CAD build for the part. Positions are in the model's coordinates, mm. A direction names the side the tool comes from. Give positions to 0.01 mm unless a question says otherwise; leave off trailing zeros. Loops run counter-clockwise (first coordinate to the right, second up) from the corner with the lowest first, then second, coordinate; pieces in that order, holes last.
```python
from build123d import *

# Parameters (mm, degrees)
SKETCH1_R                = 72.63
BOSS_EXTRUDE1_DEPTH      = 13
BOSS_EXTRUDE2_DEPTH      = 5
SKETCH4_R                = 85.63
BOSS_EXTRUDE3_DEPTH      = 3.5
BOSS_EXTRUDE3_DEPTH_BACK = 5
CUT_EXTRUDE1_DEPTH       = 6
FILLET1_R                = 50
FILLET2_R                = 5
SKETCH8_R                = 2.4
CUT_EXTRUDE2_DEPTH       = 9.5
SKETCH10_OUTSIDE_W       = 230.742
SKETCH10_OUTSIDE_H       = 289.594
SKETCH10_OUTSIDE_R       = 60
CUT_EXTRUDE3_DEPTH       = 19
SKETCH11_R               = 2.4
CUT_EXTRUDE4_DEPTH       = 19


with BuildPart() as part:
    # Sketch1 → Boss-Extrude1 (new body)
    with BuildSketch(Plane(origin=(0, 0, 0), x_dir=(1, 0, 0), z_dir=(0, 1, 0))):
        Circle(SKETCH1_R)
    extrude(amount=BOSS_EXTRUDE1_DEPTH)

    # Sketch2 → Boss-Extrude2 (add)
    with BuildSketch(Plane(origin=(0, 13, 0), x_dir=(1, 0, 0), z_dir=(0, 1, 0))):
        with BuildLine():
            Line((-21.15, -69.482331567), (-21.15, -144.482331567))
            Line((-21.15, -144.482331567), (21.15, -144.482331567))
            Line((21.15, -144.482331567), (21.15, -69.482331567))
            ThreePointArc((21.15, -69.482331567), (0, 72.63), (-21.15, -69.482331567))
        make_face()
    extrude(amount=BOSS_EXTRUDE2_DEPTH)

    # Sketch4 → Boss-Extrude3 (add, two sides)
    with BuildSketch(Plane.XZ.offset(-13)) as boss_extrude3_sk:
        Circle(SKETCH4_R)
    extrude(amount=BOSS_EXTRUDE3_DEPTH)
    extrude(boss_extrude3_sk.sketch, amount=-BOSS_EXTRUDE3_DEPTH_BACK)

    # Sketch5 → Cut-Extrude1 (cut, through all)
    with BuildSketch(Plane.XZ.offset(-13)):
        with BuildLine():
            Line((11.25, 123.332331567), (11.25, 119.332331567))
            ThreePointArc((11.25, 119.332331567), (0, 108.082331567), (-11.25, 119.332331567))
            Line((-11.25, 119.332331567), (-11.25, 123.332331567))
            ThreePointArc((-11.25, 123.332331567), (0, 134.582331567), (11.25, 123.332331567))
        make_face()
        with BuildLine():
            Line((17.05, 107.832331567), (17.05, 103.832331567))
            ThreePointArc((17.05, 103.832331567), (15.5, 102.282331567), (13.95, 103.832331567))
            Line((13.95, 103.832331567), (13.95, 107.832331567))
            ThreePointArc((13.95, 107.832331567), (15.5, 109.382331567), (17.05, 107.832331567))
        make_face()
        with BuildLine():
            Line((17.05, 138.832331567), (17.05, 134.832331567))
            ThreePointArc((17.05, 134.832331567), (15.5, 133.282331567), (13.95, 134.832331567))
            Line((13.95, 134.832331567), (13.95, 138.832331567))
            ThreePointArc((13.95, 138.832331567), (15.5, 140.382331567), (17.05, 138.832331567))
        make_face()
        with BuildLine():
            Line((-13.95, 138.832331567), (-13.95, 134.832331567))
            ThreePointArc((-13.95, 134.832331567), (-15.5, 133.282331567), (-17.05, 134.832331567))
            Line((-17.05, 134.832331567), (-17.05, 138.832331567))
            ThreePointArc((-17.05, 138.832331567), (-15.5, 140.382331567), (-13.95, 138.832331567))
        make_face()
        with BuildLine():
            Line((-13.95, 107.832331567), (-13.95, 103.832331567))
            ThreePointArc((-13.95, 103.832331567), (-15.5, 102.282331567), (-17.05, 103.832331567))
            Line((-17.05, 103.832331567), (-17.05, 107.832331567))
            ThreePointArc((-17.05, 107.832331567), (-15.5, 109.382331567), (-13.95, 107.832331567))
        make_face()
    extrude(amount=-CUT_EXTRUDE1_DEPTH, mode=Mode.SUBTRACT)

    # Fillet1
    fillet1_edges = [part.edges().sort_by_distance(p)[0] for p in [
        (-21.15, 15.5, 82.976951017),
        (21.15, 15.5, 82.976951017),
    ]]
    fillet(fillet1_edges, radius=FILLET1_R)

    # Fillet2
    fillet2_edges = [part.edges().sort_by_distance(p)[0] for p in [
        (-21.15, 15.5, 144.482331567),
        (21.15, 15.5, 144.482331567),
    ]]
    fillet(fillet2_edges, radius=FILLET2_R)

    # Sketch8 → Cut-Extrude2 (cut, through all)
    with BuildSketch(Plane.XZ.offset(-9.5)):
        with Locations((0, 78.7622)):
            Circle(SKETCH8_R)
    extrude(amount=-CUT_EXTRUDE2_DEPTH, mode=Mode.SUBTRACT)

    # Sketch10 outside → Cut-Extrude3 (cut, through all)
    with BuildSketch(Plane.XZ):
        with Locations((0, 29.426)):
            Rectangle(SKETCH10_OUTSIDE_W, SKETCH10_OUTSIDE_H)
        with Locations((0, 121.332331567)):
            Circle(SKETCH10_OUTSIDE_R, mode=Mode.SUBTRACT)
    extrude(amount=-CUT_EXTRUDE3_DEPTH, mode=Mode.SUBTRACT)

    # Sketch11 → Cut-Extrude4 (cut, through all)
    with BuildSketch(Plane.XZ):
        with Locations((-12.636876971, 67.569177035)):
            Circle(SKETCH11_R)
        with Locations((12.636876971, 67.569177035)):
            Circle(SKETCH11_R)
    extrude(amount=-CUT_EXTRUDE4_DEPTH, mode=Mode.SUBTRACT)


solid = part.part
```
1. Saw through at C-C, the plane x = -25. List the corners of the cut face in (y, z), and give its area (3 significant figures).
Responses:
outline: (0, 66.79) - (18, 66.79) - (18, 96.23) - (13, 96.23) - (13, 81.9) - (9.5, 81.9) - (9.5, 68.19) - (0, 68.19) - close
area: 213 mm2
2. Pull direction Z, two halves, no side cores. Call faces 1 (the face through (19.6, 15.5, 143.1)), 2 (the face through (-1, 9.5, 75)), 3 (the face through (-15.534, 15.465, 109.382)): released by +Z, released by -Z, zero draft, split by the parting line, or undercut.
Responses:
face 1: released by +Z
face 2: zero draft
face 3: undercut
3. Saw through at B-B, the plane z = 125. List the corners of the cut face in (x, y), and give its area (3 significant figures).
Responses:
outline: (-21.15, 13) - (-11.13, 13) - (-11.13, 18) - (-21.15, 18) - close; (11.13, 13) - (21.15, 13) - (21.15, 18) - (11.13, 18) - close
area: 100 mm2
4. Saw through at A-A, the plane x = 0. List the corners of the cut face in (y, z).
Responses:
outline: (0, 61.33) - (18, 61.33) - (18, 76.36) - (9.5, 76.36) - (9.5, 72.63) - (0, 72.63) - close; (9.5, 81.16) - (18, 81.16) - (18, 108.08) - (13, 108.08) - (13, 85.63) - (9.5, 85.63) - close; (13, 134.58) - (18, 134.58) - (18, 144.48) - (13, 144.48) - close
5. Saw through at D-D, the plane y = 11.5. List the corners of the cut face in (x, z).
Responses:
outline: (-39.36, 76.05) arc R60 ccw to (39.36, 76.05) arc R85.63 ccw to start; hole circle Ø4.8 at (-12.64, 67.57); hole circle Ø4.8 at (0, 78.76); hole circle Ø4.8 at (12.64, 67.57)
6. Drop flat-ended pins along their axis: pin 1 (14.5 mm diameter, centred on x = 5, z = 78.5, fed in from -Y); pin 2 (4.5 mm diameter, centred on y = 15.5, z = 137.5, fed in from -X); pin 3 (1.2 mm diameter, centred on y = 15.5, z = 105.5, fed in from -X); pin 4 (1.5 mm diameter, centred on x = -23.5, z = 135, fed in from +Y). Give the stop position or say it passes through.
Responses:
pin 1: stops at y = 0
pin 2: stops at x = -21.15
pin 3: stops at x = -22.28
pin 4: passes through
7. Probe line 1 along Z through (x, y) = (0, 12.5); line 2 along X through (y, z) = (16.25, 128); line 3 along Y through (x, z) = (35.5, 73). List the from-to ranges inside material, lowest first.
Responses:
line 1: z = 61.33 to 76.36, 81.16 to 85.63
line 2: x = -21.15 to -10.24, 10.24 to 21.15
line 3: y = 9.5 to 18
8. Tool access for faces 4 (the face through (0, 15, 144.482)), 5 (the face through (-21.15, 15, 127)), 6 (the face through (13.95, 15, 106)), 7 (the face through (21.15, 15, 128)): list every direction of +Z, -Z, +X, -X, +Y, -Y with a clear straight run to the whole face (end or side of a thin tool).
Responses:
face 4: +Z, +X, -X, +Y, -Y
face 5: +Z, -X, +Y, -Y
face 6: +Y, -Y
face 7: +Z, +X, +Y, -Y
